For this review, take the finished solid that the model builds, in its own axes (mm). Face numbers are marked on the shaded views. A direction names the side the tool comes from. Coordinates: 2 decimals unless noted, no trailing zeros. Order: outer loops, then holes, each group sorted by start corner. A loop starts at its lowest first (then second) coordinate and runs counter-clockwise, first axis right, second up. Notation, with made-up numbers: (-6, -7) - (32, -7) arc R31 cw to (32, 32) - close; hole circle Ø11 at (2.25, 13). An arc over 180 degrees is marked (long way). One line per item, written item: value. Start each with the question number.
(1) Consider section A-A on z = 5.25. Write out the cut boundary in (x, y), then the cut area to 3 significant figures.
(2) For the marked faces 1 and 2, list the 3-axis set-ups (+Z, -Z, +X, -X, +Y, -Y) from which the entire face can be reached by the end or side of a thin tool; tool diameter is ignored.
(3) Clearance check with flat-ended pins moving along their axes: pin 1 (1.5 mm diameter, centred on x = 34, z = 1.5, fed in from -Y); pin 2 (6 mm diameter, centred on x = 49.5, z = 4.5, fed in from -Y) (3 decimals); pin 3 (3.5 mm diameter, centred on x = 65.35, y = -22.97, fed in from +Z); pin 4 (5 mm diameter, centred on y = 69, z = 1, fed in from -X). State where each tip first meets the part, or that it passes through.
(4) To check wall thickness, follow line 1 along Y through (x, z) = (60, 2.5); line 2 along X through (y, z) = (-24, 3.25); line 3 along Y through (x, z) = (36, 8.25). State the ranges of each line that lie inside material, in increasing order.
(5) Consider section B-B on y = -36. Write out the cut boundary in (x, z), then the cut area to 3 significant figures.
(6) Consider section C-C on x = 26.5. Write out the cut boundary in (y, z), then the cut area to 3 significant figures.
Autodesk Fusion 360 part; units mm, degrees
sketch "Sketch1" plane through (0, 0, 0) normal (0, 0, 1) x (1, 0, 0)
  line L0 (59.3493, -22.9672) -> (59.3493, -47.9176)
  arc A0 (59.3493, -47.9176) -> (71.3493, -47.9176) centre (65.3493, -47.9176) ccw
  line L1 (71.3493, -47.9176) -> (71.3493, -22.9672)
  arc A1 (71.3493, -22.9672) -> (59.3493, -22.9672) centre (65.3493, -22.9672) ccw
  line L2 (65.3493, -22.9672) -> (65.3493, -47.9176) construction
  line L3 (61.4359, -18.4191) -> (12.6813, 83.5221)
  line L4 (12.6813, 83.5221) -> (13.3354, 93.4004)
  line L5 (13.3354, 93.4004) -> (20.0498, 95.3795)
  line L6 (23.6044, 93.7962) -> (53.1349, 32.0506)
  arc A2 (23.6044, 93.7962) -> (20.0498, 95.3795) centre (20.898, 92.5019) ccw
  line L7 (65.8452, -17.0002) -> (52.9015, 10.0639)
  line L8 (51.7229, 28.0498) -> (50.8208, 27.6184)
  line L9 (50.8208, 27.6184) -> (52.9015, 10.0639)
  arc A3 (51.7229, 28.0498) -> (53.1349, 32.0506) centre (50.4285, 30.7562) ccw
  point P0 (22.5016, 96.1021)
  point P1 (54.4293, 29.3442)
  dimension "d1" = 12
  dimension "d2" = 113
  dimension "d3" = 154.44
  dimension "d4" = 74
  dimension "d5" = 9.9
  dimension "d7" = 3
  dimension "d8" = 7
  dimension "d9" = 30
  dimension "d10" = 4.59
  dimension "d11" = 3
  dimension "d12" = 1
extrude "Extrude1" add sketch "Sketch1" along normal blind 10
sketch "Sketch2" plane through (0, 0, 10) normal (0, 0, 1) x (-1, 0, 0)
  line L0 (-50.8208, -27.6184) -> (-51.7229, -28.0498)
  arc A0 (-51.7229, -28.0498) -> (-53.1349, -32.0506) centre (-50.4285, -30.7562) ccw
  line L1 (-53.1349, -32.0506) -> (-23.6044, -93.7962)
  arc A1 (-23.6044, -93.7962) -> (-20.0498, -95.3795) centre (-20.898, -92.5019) ccw
  line L2 (-20.0498, -95.3795) -> (-13.3354, -93.4004)
  line L3 (-13.3354, -93.4004) -> (-12.6813, -83.5221)
  line L4 (-12.6813, -83.5221) -> (-61.4359, 18.4191)
  arc A2 (-61.4359, 18.4191) -> (-59.3493, 22.9672) centre (-65.3493, 22.9672) ccw
  line L5 (-59.3493, 22.9672) -> (-59.3493, 47.9176)
  arc A3 (-59.3493, 47.9176) -> (-71.3493, 47.9176) centre (-65.3493, 47.9176) ccw
  line L6 (-71.3493, 47.9176) -> (-71.3493, 22.9672)
  arc A4 (-71.3493, 22.9672) -> (-65.839, 16.9872) centre (-65.3493, 22.9672) ccw
  line L7 (-65.839, 16.9872) -> (-52.9015, -10.0639)
  line L8 (-52.9015, -10.0639) -> (-50.8208, -27.6184)
  circle A5 centre (-65.3493, 22.9672) radius 3
  circle A6 centre (-65.3493, 47.9176) radius 3
  dimension "d15" = 6
  dimension "d16" = 6
extrude "Extrude2" cut sketch "Sketch2" against normal blind 30 contours A5 | A6
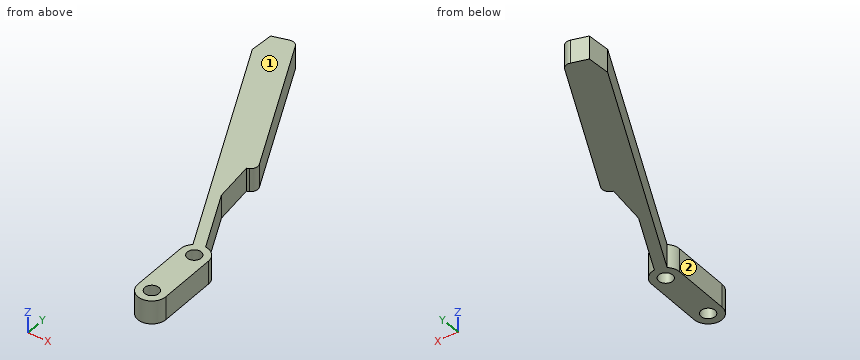
Geometry check:
1. outline: (12.68, 83.52) - (61.44, -18.42) arc R6 ccw to (59.35, -22.97) - (59.35, -47.92) arc R6 ccw to (71.35, -47.92) - (71.35, -22.97) arc R6 ccw to (65.84, -16.99) - (52.9, 10.06) - (50.82, 27.62) - (51.72, 28.05) arc R3 ccw to (53.13, 32.05) - (23.6, 93.8) arc R3 ccw to (20.05, 95.38) - (13.34, 93.4) - close; hole circle Ø6 at (65.35, -47.92); hole circle Ø6 at (65.35, -22.97)
1. area: 1,660 mm^2
2. face 1: +Z, +X, -X, +Y, -Y
2. face 2: +Z, -Z, -X, -Y
3. pin 1: stops at y = 37.38
3. pin 2: stops at y = 0.265
3. pin 3: passes through
3. pin 4: stops at x = 18.43
4. line 1: y = -50.64 to -20.25, -15.42 to -4.78
4. line 2: x = 59.35 to 62.53, 68.17 to 71.35
4. line 3: y = 34.76 to 67.88
5. outline: (59.35, 0) - (71.35, 0) - (71.35, 10) - (59.35, 10) - close
5. area: 120 mm^2
6. outline: (54.63, 0) - (87.74, 0) - (87.74, 10) - (54.63, 10) - close
6. area: 331 mm^2
